Check sheet for the drawn part. Datum: minimum x, y, z corner. Units: mm. Round coordinates to 2 decimals unless told otherwise and drop trailing zeros. Write each loop counter-clockwise with the first axis right and the second up, starting at its lowest first coordinate (ties: lowest second). Pieces come first, ordered by that corner, then holes.
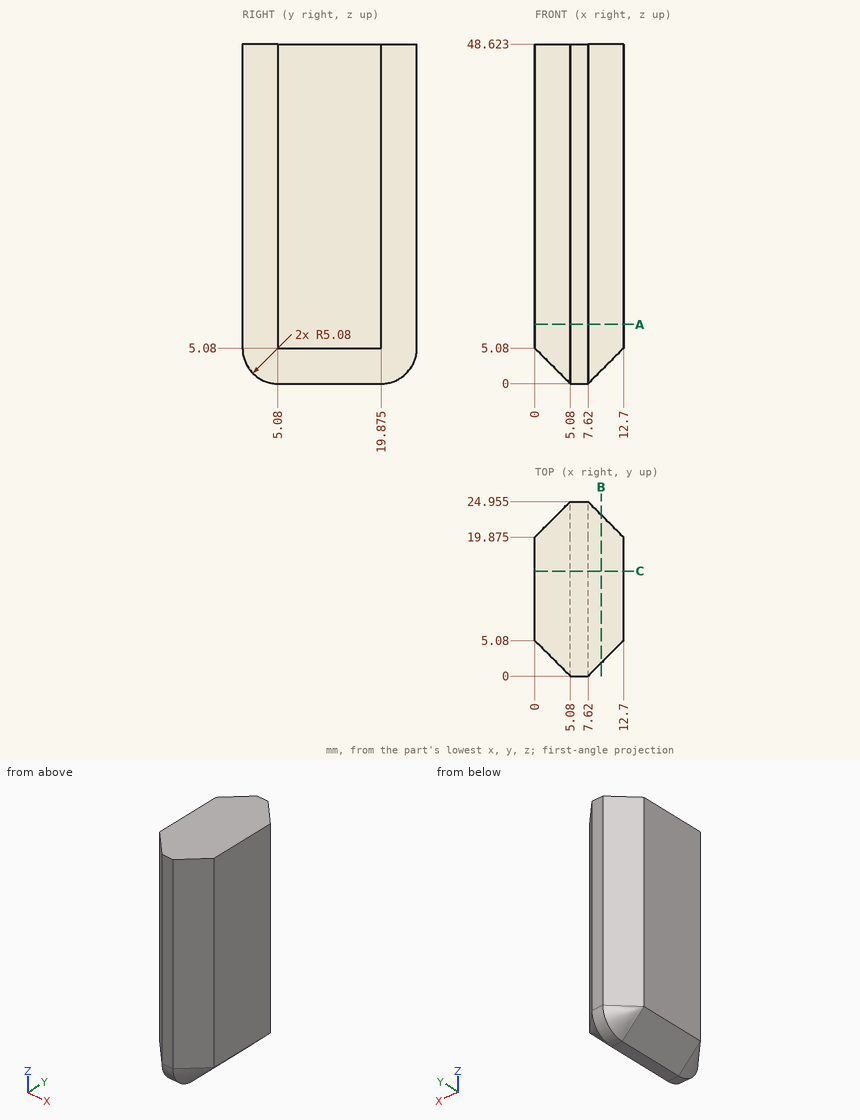
Q1. Sectioned sample at C-C (y = 15). Enter the section's corners in (x, z).
Recorded:
outline: (0, 5.08) - (5.08, 0) - (7.62, 0) - (12.7, 5.08) - (12.7, 48.62) - (0, 48.62) - close
Q2. Sectioned sample at B-B (x = 9.5). Enter the section's corners in (y, z) (1 decimal), plus the area to 3 significant figures.
Recorded:
outline: (1.9, 5.1) arc R3.2 ccw to (5.1, 1.9) - (19.9, 1.9) arc R3.2 ccw to (23.1, 5.1) - (23.1, 48.6) - (1.9, 48.6) - close
area: 986 mm2
Q3. Depth check by flat-ended pin: P1, Ø2, axis at x = 3, z = 18.5, coming from the -Y side; P2, Ø1.5, axis at y = 2.5, z = 18.5, coming from the -X side; P3, Ø5, axis at x = 8.5, y = 14, coming from the -Z side; P4, Ø2, axis at x = 3.5, z = 23.5, coming from the -Y side. Enter the tip coordinate at first touch or a pass-through.
Recorded:
P1: stops at y = 1.08
P2: stops at x = 1.83
P3: stops at z = 0
P4: stops at y = 0.58
Q4. Material ranges on line 1 along Z through (x, y) = (6.5, 3.75); line 2 along Y through (x, z) = (4.5, 38.5) (1 decimal); line 3 along Z through (x, y) = (2.25, 21) (1 decimal), recorded low to high.
Recorded:
line 1: z = 0.18 to 48.62
line 2: y = 0.6 to 24.4
line 3: z = 3.1 to 48.6
Q5. Sectioned sample at A-A (z = 8.5). Enter the section's corners in (x, y) (1 decimal).
Recorded:
outline: (0, 5.1) - (5.1, 0) - (7.6, 0) - (12.7, 5.1) - (12.7, 19.9) - (7.6, 25) - (5.1, 25) - (0, 19.9) - close
